```python
from build123d import *

# Parameters (mm, degrees)
SKETCH1_W           = 60
SKETCH1_H           = 36
BOSS_EXTRUDE1_DEPTH = 45
SHELL1_T            = -3
SKETCH2_W           = 41
SKETCH2_H           = 2
CUT_EXTRUDE1_DEPTH  = 58
SKETCH3_R           = 7.5
CUT_EXTRUDE2_DEPTH  = 48


with BuildPart() as part:
    # Sketch1 → Boss-Extrude1 (new body)
    with BuildSketch(Plane.XY):
        with Locations((30, -18)):
            Rectangle(SKETCH1_W, SKETCH1_H)
    extrude(amount=BOSS_EXTRUDE1_DEPTH)

    # Shell1
    shell1_openings = [part.faces().sort_by_distance(p)[0] for p in [
        (30, 0, 22.5),
    ]]
    offset(amount=SHELL1_T, openings=shell1_openings, kind=Kind.INTERSECTION)

    # Sketch2 → Cut-Extrude1 (cut)
    with BuildSketch(Plane(origin=(60, 0, 0), x_dir=(0, 0, -1), z_dir=(1, 0, 0))):
        with Locations((-22.5, -3)):
            Rectangle(SKETCH2_W, SKETCH2_H)
    extrude(amount=-CUT_EXTRUDE1_DEPTH, mode=Mode.SUBTRACT)

    # Sketch3 → Cut-Extrude2 (cut)
    with BuildSketch(Plane.ZY):
        with Locations(Location((22.5, -18, 0), (0, 0, 270))):
            Circle(SKETCH3_R)
    extrude(amount=-CUT_EXTRUDE2_DEPTH, mode=Mode.SUBTRACT)


solid = part.part
```
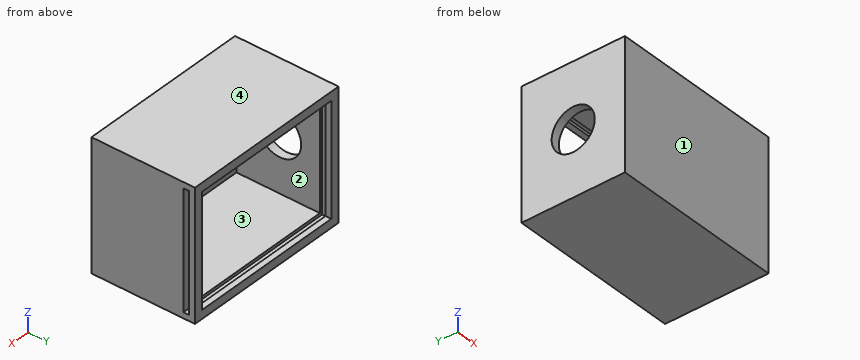
The model under review builds one solid part; all positions refer to its coordinate system, in mm. Face numbers are marked on the shaded views. Round coordinates to 2 decimals unless told otherwise and drop trailing zeros. Order: outer loops, then holes, each group sorted by start corner. A loop starts at its lowest first (then second) coordinate and runs counter-clockwise, first axis right, second up.
(1) For P1, Ø1, axis at y = -3, z = 26.5, coming from the +X side; P2, Ø2, axis at x = 31, z = 5.5, coming from the +Y side, all flat-tipped, find the tip position at first contact; note any pin that passes through.
Working result:
P1: stops at x = 2
P2: stops at y = -33
(2) Take a section at D-D, the plane z = 32.5. State the section outline as (x, y) points, plus the area to 3 significant figures.
Working result:
outline: (0, -36) - (60, -36) - (60, -4) - (57, -4) - (57, -33) - (3, -33) - (3, -4) - (2, -4) - (2, -2) - (3, -2) - (3, 0) - (0, 0) - close; (57, -2) - (60, -2) - (60, 0) - (57, 0) - close
area: 370 mm2
(3) Take a section at B-B, the plane z = 22.5. State the section outline as (x, y) points.
Working result:
outline: (0, -36) - (60, -36) - (60, -4) - (57, -4) - (57, -33) - (3, -33) - (3, -25.5) - (0, -25.5) - close; (0, -10.5) - (3, -10.5) - (3, -4) - (2, -4) - (2, -2) - (3, -2) - (3, 0) - (0, 0) - close; (57, -2) - (60, -2) - (60, 0) - (57, 0) - close
(4) Mouldability with a two-part tool opening along Z and no side actions: class the marked faces 1, 2, 3 and 4 as released by +Z, released by -Z, zero draft, split by the parting line, or undercut.
Working result:
face 1: zero draft
face 2: undercut
face 3: undercut
face 4: released by +Z
(5) Take a section at A-A, the plane y = -31. State the section outline as (x, z) points.
Working result:
outline: (0, 0) - (60, 0) - (60, 45) - (0, 45) - close; hole (3, 3) - (57, 3) - (57, 42) - (3, 42) - close
(6) Take a section at C-C, the plane x = 34.5. State the section outline as (y, z) points.
Working result:
outline: (-36, 0) - (0, 0) - (0, 3) - (-2, 3) - (-2, 2) - (-4, 2) - (-4, 3) - (-33, 3) - (-33, 42) - (-4, 42) - (-4, 43) - (-2, 43) - (-2, 42) - (0, 42) - (0, 45) - (-36, 45) - close
(7) Wall thickness on L1, parallel to X at y = -9, z = 26.5; L2, parallel to Z at x = 12, y = -26; L3, parallel to Z at x = 2.05, y = -18: over which ranges is each line inside the solid? List them lowest first.
Working result:
L1: x = 0 to 3, 57 to 60
L2: z = 0 to 3, 42 to 45
L3: z = 0 to 15, 30 to 45
